```python
from build123d import *

# Parameters (mm, degrees)
SKETCH1_R                = 82.5
BOSS_EXTRUDE1_DEPTH      = 20
SKETCH2_R                = 30
BOSS_EXTRUDE2_DEPTH      = 40
SKETCH3_R                = 17.5
CUT_EXTRUDE1_DEPTH       = 61
BOSS_EXTRUDE3_DEPTH      = 5
CIRPATTERN4_COUNT        = 3
CUT_EXTRUDE13_DEPTH      = 21
CIRPATTERN5_COUNT        = 3
CUT_EXTRUDE14_DEPTH      = 21
CIRPATTERN6_COUNT        = 3
CUT_EXTRUDE15_DEPTH      = 21
CUT_EXTRUDE15_DEPTH_BACK = 41


with BuildPart() as part:
    # Sketch1 → Boss-Extrude1 (new body)
    with BuildSketch(Plane(origin=(0, 0, 0), x_dir=(1, 0, 0), z_dir=(0, 1, 0))):
        Circle(SKETCH1_R)
    extrude(amount=BOSS_EXTRUDE1_DEPTH)

    # Sketch2 → Boss-Extrude2 (add)
    with BuildSketch(Plane.XZ):
        Circle(SKETCH2_R)
    extrude(amount=BOSS_EXTRUDE2_DEPTH)

    # Sketch3 → Cut-Extrude1 (cut, through all)
    with BuildSketch(Plane.XZ.offset(40)):
        Circle(SKETCH3_R)
    extrude(amount=-CUT_EXTRUDE1_DEPTH, mode=Mode.SUBTRACT)

    # Sketch4 → Boss-Extrude3 (add, symmetric)
    with BuildSketch(Plane.XY):
        Polygon((26.043936365, 0), (51.043936365, 0), (30, -40), (26.043936365, -40), align=None)
    boss_extrude3 = extrude(amount=BOSS_EXTRUDE3_DEPTH, both=True)

    # CirPattern4: Boss-Extrude3 ×3 about axis
    cirpattern4_axis = Axis((0, 0, 0), (0, 1, 0))
    for i in range(1, CIRPATTERN4_COUNT):
        add(boss_extrude3.rotate(cirpattern4_axis, i * 360 / CIRPATTERN4_COUNT))

    # Sketch5 → Cut-Revolve1 (revolve, cut)
    with BuildSketch(Plane.XY):
        Polygon((51.043936365, 0), (29.580398915, -40), (54.67204938, -40), align=None)
    revolve(axis=Axis((0, 0, 0), (0, -1, 0)), mode=Mode.SUBTRACT)

    # Sketch10 → Cut-Extrude13 (cut, through all)
    with BuildSketch(Plane(origin=(0, 0, 0), x_dir=(1, 0, 0), z_dir=(0, 1, 0))):
        with BuildLine():
            ThreePointArc((-60.756737715, -55.811009866), (-82.5, 0), (-60.756737715, 55.811009866))
            Line((-60.756737715, 55.811009866), (-40.932429831, 7.606987591))
            ThreePointArc((-40.932429831, 7.606987591), (-39.429287397, 0), (-40.932429831, -7.606987591))
            Line((-40.932429831, -7.606987591), (-60.756737715, -55.811009866))
        make_face()
    cut_extrude13 = extrude(amount=CUT_EXTRUDE13_DEPTH, mode=Mode.SUBTRACT)

    # CirPattern5: Cut-Extrude13 ×3 about axis
    cirpattern5_axis = Axis((0, 0, 0), (0, 1, 0))
    for i in range(1, CIRPATTERN5_COUNT):
        add(cut_extrude13.rotate(cirpattern5_axis, i * 360 / CIRPATTERN5_COUNT), mode=Mode.SUBTRACT)

    # Sketch11 → Cut-Extrude14 (cut, through all)
    with BuildSketch(Plane(origin=(0, 0, 0), x_dir=(1, 0, 0), z_dir=(0, 1, 0))):
        with BuildLine():
            Line((68.125333986, 8), (82.111205082, 8))
            ThreePointArc((82.111205082, 8), (82.5, 0), (82.111205082, -8))
            Line((82.111205082, -8), (68.125333986, -8))
            ThreePointArc((68.125333986, -8), (60.125333986, 0), (68.125333986, 8))
        make_face()
    cut_extrude14 = extrude(amount=CUT_EXTRUDE14_DEPTH, mode=Mode.SUBTRACT)

    # CirPattern6: Cut-Extrude14 ×3 about axis
    cirpattern6_axis = Axis((0, 0, 0), (0, 1, 0))
    for i in range(1, CIRPATTERN6_COUNT):
        add(cut_extrude14.rotate(cirpattern6_axis, i * 360 / CIRPATTERN6_COUNT), mode=Mode.SUBTRACT)

    # Sketch13 → Cut-Extrude15 (cut, two sides)
    with BuildSketch(Plane(origin=(0, 0, 0), x_dir=(1, 0, 0), z_dir=(0, 1, 0))) as cut_extrude15_sk:
        with BuildLine():
            Line((17.15731582, 3.446231834), (21.015929185, 3.446231834))
            Line((21.015929185, 3.446231834), (21.015929185, -3.446231834))
            Line((21.015929185, -3.446231834), (17.15731582, -3.446231834))
            ThreePointArc((17.15731582, -3.446231834), (17.5, 0), (17.15731582, 3.446231834))
        make_face()
    extrude(amount=CUT_EXTRUDE15_DEPTH, mode=Mode.SUBTRACT)
    extrude(cut_extrude15_sk.sketch, amount=-CUT_EXTRUDE15_DEPTH_BACK, mode=Mode.SUBTRACT)


solid = part.part
```
Input: part model. Units: mm. Frame: model coordinates. A direction names the side the tool comes from. Coordinates: 2 decimals unless noted, no trailing zeros. Loops run counter-clockwise (first coordinate to the right, second up) from the corner with the lowest first, then second, coordinate; pieces in that order, holes last. Notation, with made-up numbers: M 38,-19 L 43,-19 A30 ccw 43,16 Z; hole C -4.5,-7 d11. An arc over 180 degrees is marked long. Use a Markdown table: item, result. Add a question column.
1) Section C-C, the plane y = -28. Return the cut outline in (x, z).
2) Section B-B, the plane y = -17. Return the cut outline in (x, z), plus the area to 3 significant figures.
3) Set-up query: faces 5 (the flat face through (-23.32, -14.98, -30.39)), 6 (the flat face through (-44.44, 9.86, -60.97)), 7 (the flat face through (-30.68, 9.86, -69.14)). Return all of +Z, -Z, +X, -X, +Y, -Y with unobstructed straight access to the full face (end or side cutting, diameter ignored); none if empty.
4) Line query: L1, parallel to Z at x = 0, y = -23; L2, parallel to Y at x = -30, z = -25.5; L3, parallel to Z at x = 0, y = 8.5. Output: solid intervals per line, ascending. Write a range as from..to.
5) Draft query along X for faces 1 (the cylindrical face through (-54.573, 9.86, -61.871)), 2 (the flat face through (38, -15, -5)), 3 (the flat face through (19, -10, -3.446)), 4 (the cylindrical face through (19.62, 9.86, 34.2)). Return one class per face: +X half, -X half, draft (parallel to the pull), parting line (faces both ways), or undercut.
6) Pin query (flat end, axial travel): P1, Ø5, axis at y = -15, z = 1.5, coming from the +X side; P2, Ø10.5, axis at x = 37.5, y = -13.5, coming from the +Z side; P3, Ø8, axis at x = 6, z = 52, coming from the -Y side; P4, Ø2, axis at x = -45.5, z = 13.5, coming from the +Y side (1 decimal). Return the tip coordinate at first contact, or that it passes through.
7) Section A-A, the plane x = 0. Return the cut outline in (y, z), plus the area to 3 significant figures.
Answer below:
| question | item | result |
|---|---|---|
| 1 | outline | M -22.17,-28.39 A36.02 ccw -13.51,-33.39 L -10.46,-28.12 A30 ccw 29.58,-5 L 35.67,-5 A36.02 ccw 35.67,5 L 29.58,5 A30 ccw -10.46,28.12 L -13.51,33.39 A36.02 ccw -22.17,28.39 L -19.12,23.12 A30 ccw -19.12,-23.12 Z; hole M 17.16,-3.45 L 21.02,-3.45 L 21.02,3.45 L 17.16,3.45 A17.5 ccw long Z |
| 2 | outline | M -25.14,-33.55 A41.92 ccw -16.48,-38.55 L -10.46,-28.12 A30 ccw 29.58,-5 L 41.62,-5 A41.92 ccw 41.62,5 L 29.58,5 A30 ccw -10.46,28.12 L -16.48,38.55 A41.92 ccw -25.14,33.55 L -19.12,23.12 A30 ccw -19.12,-23.12 Z; hole M 17.16,-3.45 L 21.02,-3.45 L 21.02,3.45 L 17.16,3.45 A17.5 ccw long Z |
| 2 | area | 2,200 mm2 |
| 3 | face 5 | -X, -Y |
| 3 | face 6 | -Z, +Y, -Y |
| 3 | face 7 | +Y, -Y |
| 4 | L1 | -30..-17.5, 17.5..30 |
| 4 | L2 | 0..20 |
| 4 | L3 | -57.24..-17.5, 17.5..57.24 |
| 5 | face 1 | -X half |
| 5 | face 2 | draft |
| 5 | face 3 | undercut |
| 5 | face 4 | +X half |
| 6 | P1 | x = 44.31 |
| 6 | P2 | z = 5 |
| 6 | P3 | y = 0 |
| 6 | P4 | through |
| 7 | outline | M -40,-29.58 L -39.22,-30 L 0,-30 L 0,-57.24 L 20,-57.24 L 20,-17.5 L -40,-17.5 Z; M -40,17.5 L 20,17.5 L 20,57.24 L 0,57.24 L 0,30 L -39.22,30 L -40,29.58 Z |
| 7 | area | 2,590 mm2 |
